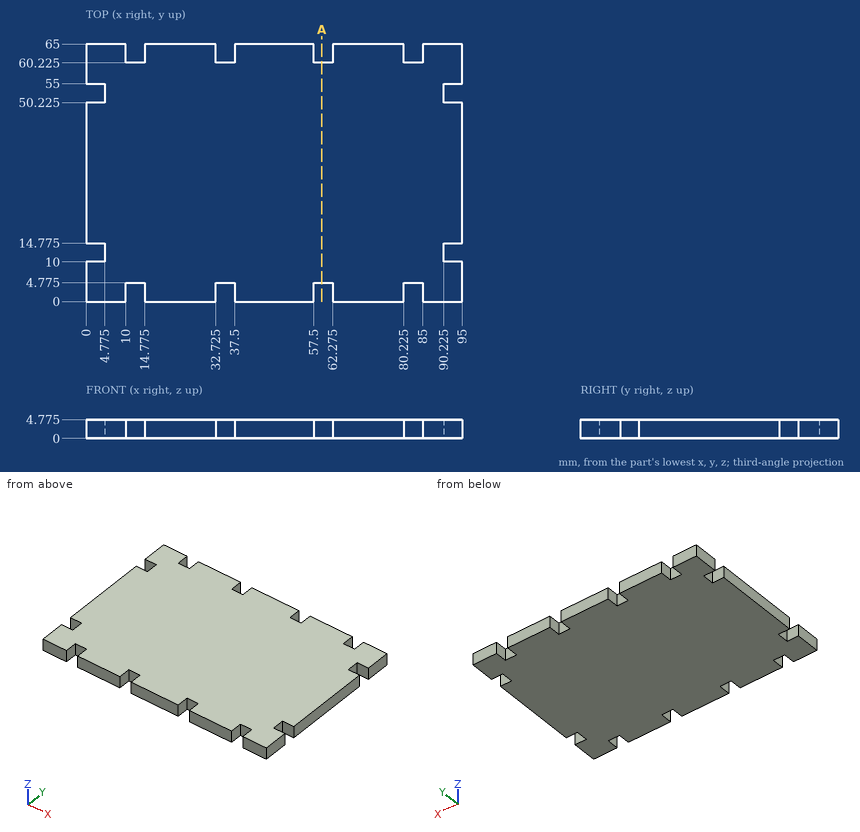
Drawing for the job (mm, zero at the part's lowest x, y, z). Coordinates: 2 decimals unless noted, no trailing zeros. Order: outer loops, then holes, each group sorted by start corner. A loop starts at its lowest first (then second) coordinate and runs counter-clockwise, first axis right, second up. Notation, with made-up numbers: (78, 86) -> (106, 86) arc R19 cw to (106, 113) -> close; hole circle Ø9 at (-29.75, 57.5). An arc over 180 degrees is marked (long way). One line per item, written item: value.
(1) Probe line 1 (X direction, y = 62.5, z = 3.5) (1 decimal); line 2 (Y direction, x = 4, z = 3.4) (1 decimal); line 3 (X direction, y = 13.5, z = 4.05) (1 decimal). List the from-to ranges inside material, lowest first. Write a range as [from, to].
Checked values:
line 1: [0, 10], [14.8, 32.7], [37.5, 57.5], [62.3, 80.2], [85, 95]
line 2: [0, 10], [14.8, 50.2], [55, 65]
line 3: [4.8, 90.2]
(2) Drop flat-ended pins along their axis: pin 1 Ø1.4 at (x, z) = (11.5, 1.5) entering from +Y (3 decimals); pin 2 Ø1.4 at (x, z) = (93.5, 3) entering from -Y; pin 3 Ø2.5 at (y, z) = (52, 2.5) entering from -X (3 decimals); pin 4 Ø1 at (x, z) = (36, 2) entering from -Y (3 decimals). Give the stop position or say it passes through.
Checked values:
pin 1: y = 60.225
pin 2: y = 0
pin 3: x = 4.775
pin 4: y = 4.775
(3) Slice it at A-A, the plane x = 59.5. List the corners of the cut face in (y, z) (1 decimal), plus the area to 3 significant figures.
Checked values:
outline: (4.8, 0) -> (60.2, 0) -> (60.2, 4.8) -> (4.8, 4.8) -> close
area: 265 mm2
